Input: part model. Units: mm. Frame: model coordinates. A direction names the side the tool comes from. Give positions to 0.01 mm unless a question says otherwise; leave off trailing zeros. Loops run counter-clockwise (first coordinate to the right, second up) from the corner with the lowest first, then second, coordinate; pieces in that order, holes last. Notation, with made-up numbers: M 59,66 L 97,66 A25 cw 97,93 Z; hole C -13,-31.5 d2. An arc over 180 degrees is marked long. Answer as a JSON object with one key per item and string values. Group by question number.
1) Draft query along Y for faces 3 (the flat face through (0, -2, 0)), 4 (the cylindrical face through (2.465, -1.082, 7.414)). Return one class per face: +Y half, -Y half, draft (parallel to the pull), parting line (faces both ways), or undercut.
2) Ray query, L1, parallel to Z at x = 0.6, y = 0; L2, parallel to Y at x = 4.3, z = 6.25; L3, parallel to X at y = 4, z = -4.25. Return the intervals inside material, ascending.
3) Section query C-C on z = 4.5. Return loops of the section in (x, y).
4) Section query A-A on y = -7.5. Return loops of the section in (x, z).
5) First-contact query: P1, Ø1, axis at x = 1, z = -6.5, coming from the -Y side; P2, Ø2, axis at x = 2, y = 4, coming from the -Z side; P3, Ø1.8, axis at y = 0, z = 0, coming from the +X side. Flat tips, straight axial feed; report the tip coordinate or a pass-through.
6) Section query B-B on y = -3. Return loops of the section in (x, z).
7) Access query for faces 1 (the flat face through (5, -2, 0)), 2 (the flat face through (4.39, 0.77, -0.58)). Directions: +Z, -Z, +X, -X, +Y, -Y. A direction counts if a zero-diameter tool reaches every point of the face in a straight line with its end or side. Return the directions, or none.
from build123d import *

# Parameters (mm, degrees)
BASPROSKE_W         = 5
BASPROSKE_H         = 9
TOOTHCUT_DEPTH      = 14.674794331
TEETHCUTS_COUNT     = 10
TEETHCUTS_ANGLE     = 324
BORSKE_R            = 1.5
BORE_DEPTH          = 50.0001524
EXTRUDE_1_DEPTH     = 5
SKETCH_3_R          = 1.5
CUT_EXTRUDE_1_DEPTH = 7


with BuildPart() as part:
    # BasProSke → Base-Revolve (revolve)
    with BuildSketch(Plane(origin=(0, 0, 0), x_dir=(1, 0, 0), z_dir=(0, 1, 0)), mode=Mode.PRIVATE) as base_revolve_sk:
        with Locations((2.5, 4.5)):
            Rectangle(BASPROSKE_W, BASPROSKE_H)
    revolve(base_revolve_sk.sketch.rotate(Axis((-10, 0, 0), (1, 0, 0)), 180), axis=Axis((-10, 0, 0), (1, 0, 0)))

    # TooCutSke → ToothCut (cut, through all)
    with BuildSketch(Plane(origin=(0, 0, 0), x_dir=(0, 0, -1), z_dir=(1, 0, 0))):
        with BuildLine():
            ThreePointArc((0.883878355, 5.554109745), (0, 5.624), (-0.883878355, 5.554109745))
            ThreePointArc((-0.883878355, 5.554109745), (-1.258245767, 7.379188248), (-2.637816971, 8.631324741))
            ThreePointArc((-2.637816971, 8.631324741), (0, 9.0254), (2.637816971, 8.631324741))
            ThreePointArc((2.637816971, 8.631324741), (1.258245767, 7.379188248), (0.883878355, 5.554109745))
        make_face()
    toothcut = extrude(amount=TOOTHCUT_DEPTH, mode=Mode.SUBTRACT)

    # TeethCuts: ToothCut ×10 about axis
    teethcuts_axis = Axis((-10, 0, 0), (1, 0, 0))
    for i in range(1, TEETHCUTS_COUNT):
        add(toothcut.rotate(teethcuts_axis, i * TEETHCUTS_ANGLE / (TEETHCUTS_COUNT - 1)), mode=Mode.SUBTRACT)

    # BorSke → Bore (cut, symmetric)
    with BuildSketch(Plane(origin=(0, 0, 0), x_dir=(0, 0, -1), z_dir=(1, 0, 0))):
        with Locations(Location((0, 0, 0), (0, 0, 180))):
            Circle(BORSKE_R)
    extrude(amount=BORE_DEPTH, both=True, mode=Mode.SUBTRACT)

    # 草圖2 → 填料-伸長1 (add, through all)
    with BuildSketch(Plane(origin=(0, 0, 0), x_dir=(0, 0, -1), z_dir=(1, 0, 0))):
        with BuildLine():
            ThreePointArc((-0.364292368, 1.45509143), (0.881677878, 1.213525492), (1.496446719, 0.10318535))
            Line((1.496446719, 0.10318535), (-0.364292368, 1.45509143))
        make_face()
    extrude(amount=EXTRUDE_1_DEPTH)

    # 草圖3 → 除料-伸長1 (cut)
    with BuildSketch(Plane(origin=(0, 0.77913839, -0.566077176), x_dir=(1, 0, 0), z_dir=(0, -0.8090169943749549, 0.5877852522924627))):
        with Locations(Location((2.5, 0, 0), (0, 0, 230.05549481))):
            Circle(SKETCH_3_R)
    extrude(amount=-CUT_EXTRUDE_1_DEPTH, mode=Mode.SUBTRACT)


solid = part.part
Output:
{
 "1": {"face 3": "draft", "face 4": "undercut"},
 "2": {"L1": "z = -9 to -1.5, 1.5 to 9", "L2": "y = -5.48 to -3.13, -1.1 to 1.1, 3.13 to 5.48", "L3": "x = 0 to 1.47, 3.53 to 5"},
 "3": {"outline": "M 0,-4.65 L 5,-4.65 L 5,4.65 L 0,4.65 Z"},
 "4": {"outline": "M 0,-3.3 L 5,-3.3 L 5,-1.33 L 0,-1.33 Z; M 0,1.33 L 5,1.33 L 5,3.3 L 0,3.3 Z"},
 "5": {"P1": "stops at y = -5.5", "P2": "stops at z = -7.37", "P3": "passes through"},
 "6": {"outline": "M 0,-6.07 L 5,-6.07 L 5,6.07 L 0,6.07 Z"},
 "7": {"face 1": "+Z, -Z, +X, +Y, -Y", "face 2": "+X, -X"}
}
